Geometry check sheet. Reference: the model listing, model coordinates, mm. Round coordinates to 2 decimals unless told otherwise and drop trailing zeros. Write each loop counter-clockwise with the first axis right and the second up, starting at its lowest first coordinate (ties: lowest second). Pieces come first, ordered by that corner, then holes. Notation, with made-up numbers: M 55.5,89 L 96.5,89 A28 cw 96.5,121 Z; hole C -21.5,80.25 d7. An arc over 180 degrees is marked long. One line per item, written item: value. Start each with the question number.
1. Depth check by flat-ended pin: P1, Ø3, axis at x = -77, z = -296, coming from the +Y side; P2, Ø2, axis at x = -174, z = -168, coming from the +Y side; P3, Ø4, axis at x = -354.5, z = -391.5, coming from the +Y side. Enter the tip coordinate at first touch or a pass-through.
2. Scan lines: probe 1 along Y at (x, z) = (-1, -496.5); probe 2 along Y at (x, z) = (-264.5, -408.5). Record each from-to range of solid material in increasing order. Write a range as [from, to].
3. Section check A-A (z = -459). Record the boundary of the cut face in (x, y).
4. Section check B-B (x = -262.5). Record the boundary of the cut face in (y, z), and give its area (3 significant figures).
from build123d import *

# Parameters (mm, degrees)
BOSS_EXTRUDE1_DEPTH     = 2
SKETCH3_R               = 4.1
CUT_EXTRUDE1_DEPTH      = 150
MIRROR2_COPY_1_SKETCH_R = 4.1
MIRROR2_COPY_1_DEPTH    = 150


with BuildPart() as part:
    # Sketch2 → Boss-Extrude1 (new body)
    with BuildSketch(Plane(origin=(75.209264803, -1945.500458031, -70.562482719), x_dir=(0.9992543484228519, 0.038603856587709914, 0.0006995817159617483), z_dir=(-0.03860385658770992, 0.998597990155389, 0.03621872877633121))):
        with BuildLine():
            Line((-488.860391094, 45.687428375), (-68.860391094, 45.687428375))
            ThreePointArc((-68.860391094, 45.687428375), (-61.789323282, 48.616360563), (-58.860391094, 55.687428375))
            Line((-58.860391094, 55.687428375), (-58.860391094, 475.687428375))
            ThreePointArc((-58.860391094, 475.687428375), (-61.789323282, 482.758496187), (-68.860391094, 485.687428375))
            Line((-68.860391094, 485.687428375), (-488.860391094, 485.687428375))
            ThreePointArc((-488.860391094, 485.687428375), (-495.931458906, 482.758496187), (-498.860391094, 475.687428375))
            Line((-498.860391094, 475.687428375), (-498.860391094, 55.687428375))
            ThreePointArc((-498.860391094, 55.687428375), (-495.931458906, 48.616360563), (-488.860391094, 45.687428375))
        make_face()
    extrude(amount=BOSS_EXTRUDE1_DEPTH)

    # Sketch3 → Cut-Extrude1 (cut)
    with BuildSketch(Plane(origin=(-103.287183068, -1885.761116085, -334.134352796), x_dir=(-0.0006995817159619569, 0.036218728776338416, -0.9993436417325368), z_dir=(0.038603856587716694, -0.9985979901553884, -0.036218728776338416))):
        with Locations(Location((-203.071067812, 100.352249502, 0), (0, 0, 269.959890601))):
            Circle(SKETCH3_R)
    cut_extrude1 = extrude(amount=CUT_EXTRUDE1_DEPTH, mode=Mode.SUBTRACT)

    # Mirror1: Cut-Extrude1 across plane
    add(cut_extrude1.mirror(Plane(origin=(-278.652458404, -10.765086546, -0.195085631), x_dir=(-0.000699060242817171, -2.700655884307846e-05, 0.9999997552926815), z_dir=(-0.9992543484228519, -0.03860385658770997, -0.0006995817159618643))), mode=Mode.SUBTRACT)

    # Mirror2: Cut-Extrude1 across plane
    add(cut_extrude1.mirror(Plane(origin=(-0.185870067, 9.622860908, -265.513042235), x_dir=(0.9999997552926815, 2.5337966627687505e-05, -0.0006991227107992283), z_dir=(0.0006995817159618217, -0.036218728776331255, 0.9993436417325371))), mode=Mode.SUBTRACT)

    # Mirror2 copy 1 sketch → Mirror2 copy 1 (cut)
    with BuildSketch(Plane(origin=(-308.371783919, -1893.684080376, -334.277933294), x_dir=(0.0006995817159616872, -0.0362187287763241, 0.9993436417325376), z_dir=(0.03860385658770326, -0.9985979901553895, -0.0362187287763241))):
        with Locations(Location((-203.071067812, 100.352249502, 0), (0, 0, 269.959890601))):
            Circle(MIRROR2_COPY_1_SKETCH_R)
    extrude(amount=MIRROR2_COPY_1_DEPTH, mode=Mode.SUBTRACT)


solid = part.part
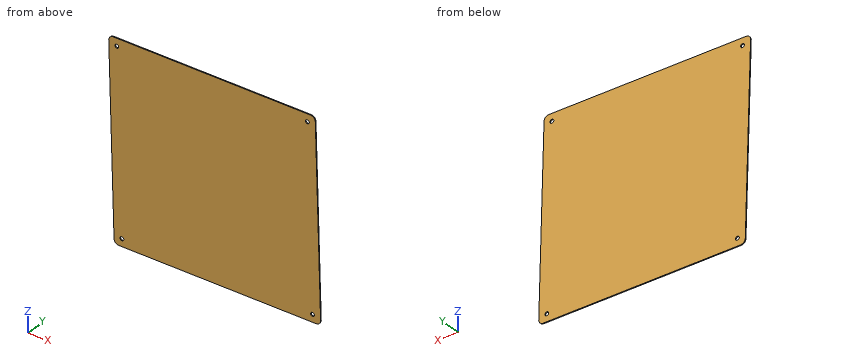
Result sheet:
1. P1: stops at y = -1941.13
1. P2: stops at y = -1949.54
1. P3: stops at y = -1948.36
2. probe 1: y = [-1933, -1931]
2. probe 2: y = [-1946.38, -1944.37]
3. outline: M -423.63,-1948.69 L -423.55,-1950.69 L 16.12,-1933.7 L 16.04,-1931.7 Z
4. outline: M -1956.89,-116.46 L -1940.94,-556.17 L -1938.94,-556.09 L -1954.89,-116.38 Z
4. area: 881 mm2
